Here's the drawing with two shaded views (mm, measured from the low corner). I have some questions. Round coordinates to 2 decimals unless told otherwise and drop trailing zeros. Order: outer loops, then holes, each group sorted by start corner. A loop starts at its lowest first (then second) coordinate and runs counter-clockwise, first axis right, second up.
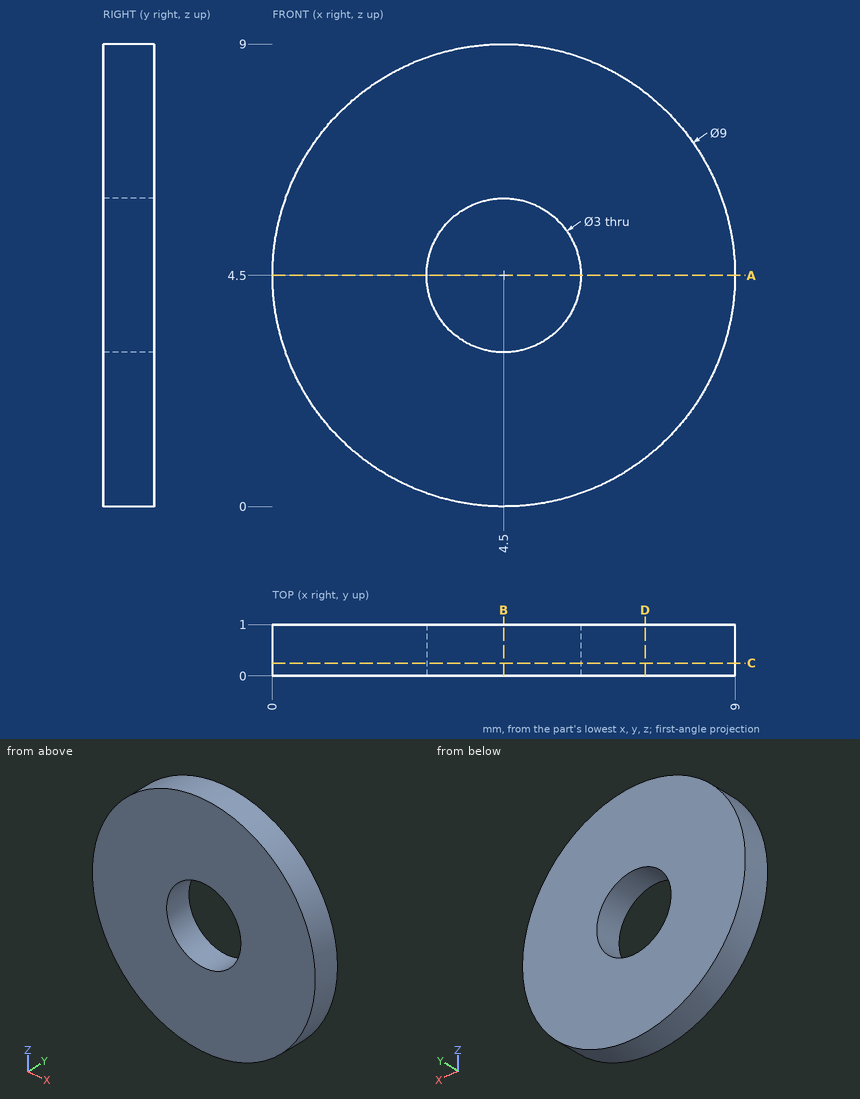
1. If we section it at B-B, the plane x = 4.5: Write out the boundary of the cut face in (y, z).
Evaluation:
outline: (0, 0) - (1, 0) - (1, 3) - (0, 3) - close; (0, 6) - (1, 6) - (1, 9) - (0, 9) - close
2. If we section it at D-D, the plane x = 7.25: Write out the boundary of the cut face in (y, z).
Evaluation:
outline: (0, 0.94) - (1, 0.94) - (1, 8.06) - (0, 8.06) - close
3. If we section it at A-A, the plane z = 4.5: Write out the boundary of the cut face in (x, y), and give its area (3 significant figures).
Evaluation:
outline: (0, 0) - (3, 0) - (3, 1) - (0, 1) - close; (6, 0) - (9, 0) - (9, 1) - (6, 1) - close
area: 6.00 mm2
4. I need wall thicknesses on probe 1 along X at (y, z) = (0.4, 4.5); probe 2 along Z at (x, y) = (3.75, 0.3). Which ranges of each line are inside material? Lowest first, please.
Evaluation:
probe 1: x = 0 to 3, 6 to 9
probe 2: z = 0.06 to 3.2, 5.8 to 8.94
5. If we section it at C-C, the plane y = 0.25: Write out the boundary of the cut face in (x, z).
Evaluation:
outline: circle Ø9 at (4.5, 4.5); hole circle Ø3 at (4.5, 4.5)
